Design review of the part shown in the three views and the two pictorial views. Dimensions are in mm from the part's minimum x, y and z. A direction names the side the tool comes from. Give positions to 0.01 mm unless a question says otherwise; leave off trailing zeros. Order: outer loops, then holes, each group sorted by start corner. A loop starts at its lowest first (then second) coordinate and runs counter-clockwise, first axis right, second up. Notation, with made-up numbers: (9.5, -36) - (34.5, -36) arc R22 ccw to (34.5, -21) - close; hole circle Ø4 at (4.25, -37). An arc over 180 degrees is marked (long way). Put each result on its own line as item: value.
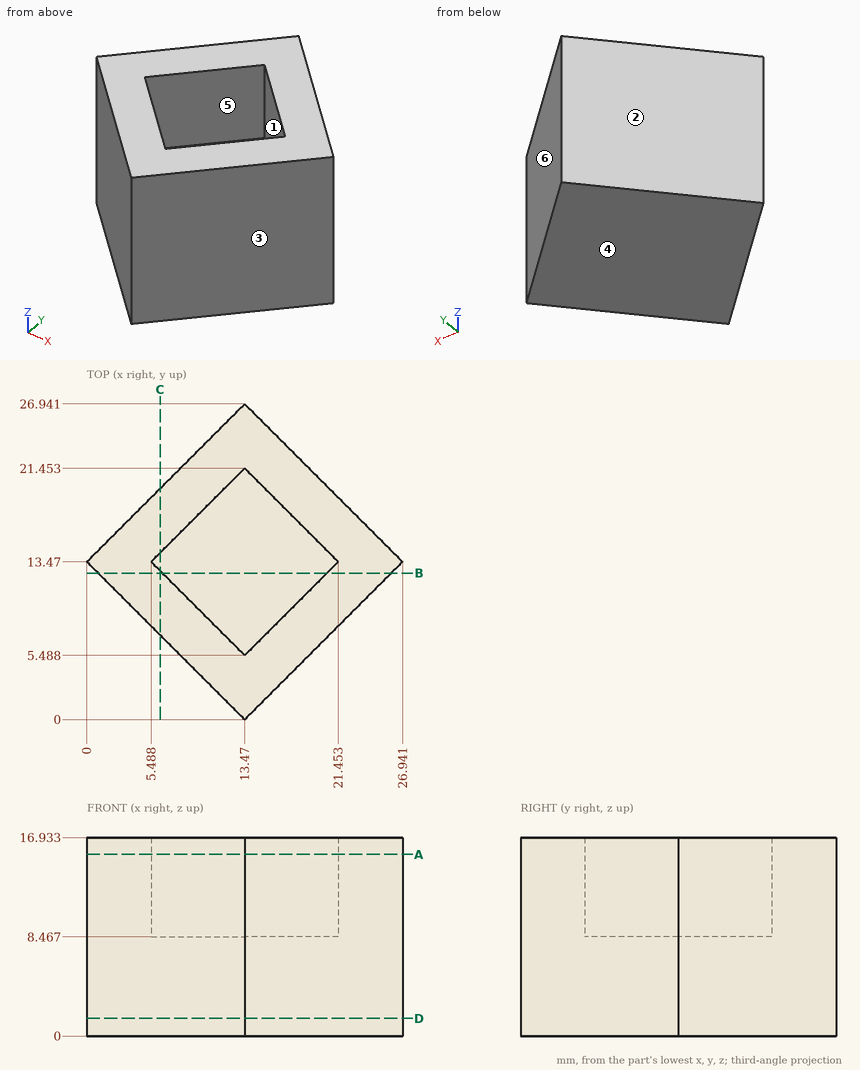
(1) For the marked faces 5 and 6, list the 3-axis set-ups (+Z, -Z, +X, -X, +Y, -Y) from which the entire face can be reached by the end or side of a thin tool; tool diameter is ignored.
The answers:
face 5: +Z
face 6: +Z, -Z, +X, +Y
(2) Take a section at A-A, the plane z = 15.5. Write out the cut boundary in (x, y).
The answers:
outline: (0, 13.47) - (13.47, 0) - (26.94, 13.47) - (13.47, 26.94) - close; hole (5.49, 13.47) - (13.47, 5.49) - (21.45, 13.47) - (13.47, 21.45) - close
(3) Take a section at C-C, the plane x = 6.25. Write out the cut boundary in (y, z).
The answers:
outline: (7.22, 0) - (19.72, 0) - (19.72, 16.93) - (14.23, 16.93) - (14.23, 8.47) - (12.71, 8.47) - (12.71, 16.93) - (7.22, 16.93) - close
(4) Take a section at D-D, the plane z = 1.5. Write out the cut boundary in (x, y), then the cut area to 3 significant figures.
The answers:
outline: (0, 13.47) - (13.47, 0) - (26.94, 13.47) - (13.47, 26.94) - close
area: 363 mm^2
(5) The part is to be moulded in two halves that separate along Y. For the marked faces 1, 2, 3 and 4, say which applies: pulls with the +Y half, pulls with the -Y half, needs draft (parallel to the pull), parting line crosses it, or undercut.
The answers:
face 1: undercut
face 2: pulls with the +Y half
face 3: pulls with the -Y half
face 4: needs draft
(6) Clearance check with flat-ended pins moving along their axes: pin 1 Ø4 at (x, z) = (18.5, 15) entering from +Y; pin 2 Ø4 at (y, z) = (20, 5.5) entering from -X; pin 3 Ø1 at (x, z) = (23.5, 9.5) entering from +Y. State where each tip first meets the part, or that it passes through.
The answers:
pin 1: y = 23.91
pin 2: x = 4.53
pin 3: y = 17.41
(7) Take a section at B-B, the plane y = 12.5. Write out the cut boundary in (x, z).
The answers:
outline: (0.97, 0) - (25.97, 0) - (25.97, 16.93) - (20.48, 16.93) - (20.48, 8.47) - (6.46, 8.47) - (6.46, 16.93) - (0.97, 16.93) - close
(8) Wall thickness on L1, parallel to X at y = 14.5, z = 9.5 (1 decimal); L2, parallel to X at y = 8.5, z = 14.75; L3, parallel to Z at x = 6, y = 13.25: over which ranges is each line inside the solid? List them lowest first.
The answers:
L1: 1 to 6.5, 20.4 to 25.9
L2: 4.97 to 10.46, 16.48 to 21.97
L3: 0 to 8.47
